```python
from build123d import *

# Parameters (mm, degrees)
F0_R     = 10
F1_DEPTH = 40
F2_DEPTH = 30


with BuildPart() as f1:
    # F0 (on Top) → F1 (new body, symmetric)
    with BuildSketch(Plane.XY):
        with BuildLine():
            Line((75, 35), (-75, 35))
            ThreePointArc((-75, 35), (-110, 0), (-75, -35))
            Line((-75, -35), (75, -35))
            ThreePointArc((75, -35), (110, 0), (75, 35))
        make_face()
        with BuildLine():
            ThreePointArc((-42.5, 0), (-75, -32.5), (-107.5, 0))
            Line((-107.5, 0), (-86.25, 0))
            ThreePointArc((-86.25, 0), (-75, 11.25), (-63.75, 0))
            Line((-63.75, 0), (-42.5, 0))
        make_face(mode=Mode.SUBTRACT)
        with BuildLine():
            ThreePointArc((107.5, 0), (75, -32.5), (42.5, 0))
            Line((42.5, 0), (63.75, 0))
            ThreePointArc((63.75, 0), (75, 11.25), (86.25, 0))
            Line((86.25, 0), (107.5, 0))
        make_face(mode=Mode.SUBTRACT)
        Circle(F0_R, mode=Mode.SUBTRACT)
        with BuildLine():
            Line((-86.25, 0), (-107.5, 0))
            ThreePointArc((-107.5, 0), (-75, -32.5), (-42.5, 0))
            Line((-42.5, 0), (-63.75, 0))
            ThreePointArc((-63.75, 0), (-75, -11.25), (-86.25, 0))
        make_face()
        with BuildLine():
            Line((63.75, 0), (42.5, 0))
            ThreePointArc((42.5, 0), (75, -32.5), (107.5, 0))
            Line((107.5, 0), (86.25, 0))
            ThreePointArc((86.25, 0), (75, -11.25), (63.75, 0))
        make_face()
        Circle(F0_R)
    extrude(amount=F1_DEPTH, both=True)

    # F0 (on Top) → F2 (cut, symmetric)
    with BuildSketch(Plane.XY):
        with BuildLine():
            Line((75, 35), (-75, 35))
            ThreePointArc((-75, 35), (-110, 0), (-75, -35))
            Line((-75, -35), (75, -35))
            ThreePointArc((75, -35), (110, 0), (75, 35))
        make_face()
        with BuildLine():
            ThreePointArc((-42.5, 0), (-75, -32.5), (-107.5, 0))
            Line((-107.5, 0), (-86.25, 0))
            ThreePointArc((-86.25, 0), (-75, 11.25), (-63.75, 0))
            Line((-63.75, 0), (-42.5, 0))
        make_face(mode=Mode.SUBTRACT)
        with BuildLine():
            ThreePointArc((107.5, 0), (75, -32.5), (42.5, 0))
            Line((42.5, 0), (63.75, 0))
            ThreePointArc((63.75, 0), (75, 11.25), (86.25, 0))
            Line((86.25, 0), (107.5, 0))
        make_face(mode=Mode.SUBTRACT)
        Circle(F0_R, mode=Mode.SUBTRACT)
        with BuildLine():
            Line((-86.25, 0), (-107.5, 0))
            ThreePointArc((-107.5, 0), (-75, -32.5), (-42.5, 0))
            Line((-42.5, 0), (-63.75, 0))
            ThreePointArc((-63.75, 0), (-75, -11.25), (-86.25, 0))
        make_face()
        with BuildLine():
            Line((63.75, 0), (42.5, 0))
            ThreePointArc((42.5, 0), (75, -32.5), (107.5, 0))
            Line((107.5, 0), (86.25, 0))
            ThreePointArc((86.25, 0), (75, -11.25), (63.75, 0))
        make_face()
    extrude(amount=F2_DEPTH, both=True, mode=Mode.SUBTRACT)


solid = f1.part
```
Can you work these out from the model? Positions are in its coordinate system, mm. A direction names the side the tool comes from. Coordinates: 2 decimals unless noted, no trailing zeros. Loops run counter-clockwise (first coordinate to the right, second up) from the corner with the lowest first, then second, coordinate; pieces in that order, holes last.
1) Which directions (+Z, -Z, +X, -X, +Y, -Y) give clear straight access to the entire face, cutting with the end or side of a thin tool? Please do faces 4 (the cylindrical face through (-2.17, -9.76, 0.42)), 5 (the flat face through (-1, -35, 35)).
2) Imagine slicing it at C-C on y = -19.5. List the corners of the cut face in (x, z) for me, plus the area to 3 significant figures.
3) Imagine slicing it at B-B on x = -16. List the corners of the cut face in (y, z) for me, plus the area to 3 significant figures.
4) Imagine slicing it at A-A on y = 0. List the corners of the cut face in (x, z) for me.
5) I need wall thicknesses on probe 1 along Z at (x, y) = (39, -24); probe 2 along Y at (x, z) = (75, 37.5); probe 3 along X at (y, z) = (-4.5, -35). Which ranges of each line are inside material? Lowest first, please.
6) For pin 1 (1.5 mm diameter, centred on y = -1, z = -32, fed in from -X), with a flat end and sliding along its axis, tell me the tip position at first contact or that it passes through.
7) Thinking about a two-plate mould opening in Y: for faces 1 (the cylindrical face through (-109.99, 0.77, -34.93)), 2 (the cylindrical face through (-64.27, -3.38, 35.07)), 3 (the flat face through (-1, -35, -35)), which applies, pulls with the +Y half, pulls with the -Y half, needs draft (parallel to the pull), parting line crosses it, or undercut?
8) Imagine slicing it at D-D on x = 81.5. List the corners of the cut face in (y, z) for me.
Completed:
1. face 4: none
1. face 5: +Z, -Z, +X, -X, -Y
2. outline: (-104.06, -40) - (104.06, -40) - (104.06, -30) - (-104.06, -30) - close; (-104.06, 30) - (104.06, 30) - (104.06, 40) - (-104.06, 40) - close
2. area: 4,160 mm2
3. outline: (-35, -40) - (35, -40) - (35, -30) - (-35, -30) - close; (-35, 30) - (35, 30) - (35, 40) - (-35, 40) - close
3. area: 1,400 mm2
4. outline: (-110, -40) - (-86.25, -40) - (-86.25, -30) - (-110, -30) - close; (-110, 30) - (-86.25, 30) - (-86.25, 40) - (-110, 40) - close; (-63.75, -40) - (63.75, -40) - (63.75, -30) - (10, -30) - (10, 30) - (63.75, 30) - (63.75, 40) - (-63.75, 40) - (-63.75, 30) - (-10, 30) - (-10, -30) - (-63.75, -30) - close; (86.25, -40) - (110, -40) - (110, -30) - (86.25, -30) - close; (86.25, 30) - (110, 30) - (110, 40) - (86.25, 40) - close
5. probe 1: z = -40 to -30, 30 to 40
5. probe 2: y = -35 to -11.25, 11.25 to 35
5. probe 3: x = -109.71 to -85.31, -64.69 to 64.69, 85.31 to 109.71
6. pin 1: stops at x = -110
7. face 1: parting line crosses it
7. face 2: undercut
7. face 3: pulls with the -Y half
8. outline: (-34.39, -40) - (-9.18, -40) - (-9.18, -30) - (-34.39, -30) - close; (-34.39, 30) - (-9.18, 30) - (-9.18, 40) - (-34.39, 40) - close; (9.18, -40) - (34.39, -40) - (34.39, -30) - (9.18, -30) - close; (9.18, 30) - (34.39, 30) - (34.39, 40) - (9.18, 40) - close
